CAD build for the part. Positions are in the model's coordinates, mm. Give positions to 0.01 mm unless a question says otherwise; leave off trailing zeros. Loops run counter-clockwise (first coordinate to the right, second up) from the corner with the lowest first, then second, coordinate; pieces in that order, holes last.
```python
from build123d import *

# Parameters (mm, degrees)
SKETCH1_W           = 15
SKETCH1_H           = 15
BOSS_EXTRUDE1_DEPTH = 63
SKETCH3_R           = 1
CUT_EXTRUDE1_DEPTH  = 15
FILLET1_RADIUS      = 7.5
FILLET1_LENGTH      = 15
FILLET2_RADIUS      = 7.5
FILLET2_LENGTH      = 15


with BuildPart() as part:
    # Sketch1 → Boss-Extrude1 (new body)
    with BuildSketch(Plane(origin=(0, 0, 0), x_dir=(1, 0, 0), z_dir=(0, 1, 0))):
        Rectangle(SKETCH1_W, SKETCH1_H)
    extrude(amount=BOSS_EXTRUDE1_DEPTH)

    # Sketch3 → Cut-Extrude1 (cut)
    with BuildSketch(Plane(origin=(7.5, 0, 0), x_dir=(0, 0, -1), z_dir=(1, 0, 0))):
        with Locations((0, 59.5)):
            Circle(SKETCH3_R)
        with Locations((0, 3.5)):
            Circle(SKETCH3_R)
    extrude(amount=-CUT_EXTRUDE1_DEPTH, mode=Mode.SUBTRACT)

    # Fillet1: full round fillet: the end face becomes a half cylinder, R = half its width
    fillet1_face = Plane((0, 63, 0), x_dir=(1, 0, 0), z_dir=(0, 1, 0))  # on the end face: x along it, z out of the body
    fillet1_slab = fillet1_face.offset(-FILLET1_RADIUS / 2) * Box(FILLET1_LENGTH, 2 * FILLET1_RADIUS, FILLET1_RADIUS, mode=Mode.PRIVATE)  # the body's end, R deep
    fillet1_round = Plane((0, 55.5, 0), x_dir=(0, 1, 0), z_dir=(1, 0, 0)) * Cylinder(FILLET1_RADIUS, FILLET1_LENGTH, mode=Mode.PRIVATE)  # its axis R under the face
    add(fillet1_slab - fillet1_round, mode=Mode.SUBTRACT)

    # Fillet2: full round fillet: the end face becomes a half cylinder, R = half its width
    fillet2_face = Plane((0, 0, 0), x_dir=(-1, 0, 0), z_dir=(0, -1, 0))  # on the end face: x along it, z out of the body
    fillet2_slab = fillet2_face.offset(-FILLET2_RADIUS / 2) * Box(FILLET2_LENGTH, 2 * FILLET2_RADIUS, FILLET2_RADIUS, mode=Mode.PRIVATE)  # the body's end, R deep
    fillet2_round = Plane((0, 7.5, 0), x_dir=(0, -1, 0), z_dir=(-1, 0, 0)) * Cylinder(FILLET2_RADIUS, FILLET2_LENGTH, mode=Mode.PRIVATE)  # its axis R under the face
    add(fillet2_slab - fillet2_round, mode=Mode.SUBTRACT)


solid = part.part
```
1. Drop a flat-ended pin along its axis: pin 1 (6 mm diameter, centred on x = 3.5, z = -4.5, fed in from -Y). Give the stop position or say it passes through.
Responses:
pin 1: stops at y = 0.15
2. Saw through at B-B, the plane x = -0.25. List the corners of the cut face in (y, z).
Responses:
outline: (7.5, -7.5) - (55.5, -7.5) arc R7.5 ccw to (55.5, 7.5) - (7.5, 7.5) arc R7.5 ccw to start; hole circle Ø2 at (3.5, 0); hole circle Ø2 at (59.5, 0)
3. Saw through at D-D, the plane z = 5.75. List the corners of the cut face in (x, y).
Responses:
outline: (-7.5, 2.68) - (7.5, 2.68) - (7.5, 60.32) - (-7.5, 60.32) - close
4. Saw through at A-A, the plane z = 0. List the corners of the cut face in (x, y).
Responses:
outline: (-7.5, 0) - (7.5, 0) - (7.5, 2.5) - (-7.5, 2.5) - close; (-7.5, 4.5) - (7.5, 4.5) - (7.5, 58.5) - (-7.5, 58.5) - close; (-7.5, 60.5) - (7.5, 60.5) - (7.5, 63) - (-7.5, 63) - close
5. Pull direction Z, two halves, no side cores. Call faces 1 (the face through (0.11, 4.49, 0.13)), 2 (the face through (0, 31, -7.5)), 3 (the face through (7.5, 31, 0)): released by +Z, released by -Z, zero draft, split by the parting line, or undercut.
Responses:
face 1: undercut
face 2: released by -Z
face 3: zero draft
6. Probe line 1 along Y through (x, z) = (2.75, 0); line 2 along Y through (x, z) = (-4.75, -6.25); line 3 along Y through (x, z) = (-3.75, -4.5). List the from-to ranges inside material, lowest first.
Responses:
line 1: y = 0 to 2.5, 4.5 to 58.5, 60.5 to 63
line 2: y = 3.35 to 59.65
line 3: y = 1.5 to 61.5
7. Saw through at C-C, the plane y = 3.5. List the corners of the cut face in (x, z).
Responses:
outline: (-7.5, -6.34) - (7.5, -6.34) - (7.5, -1) - (-7.5, -1) - close; (-7.5, 1) - (7.5, 1) - (7.5, 6.34) - (-7.5, 6.34) - close
